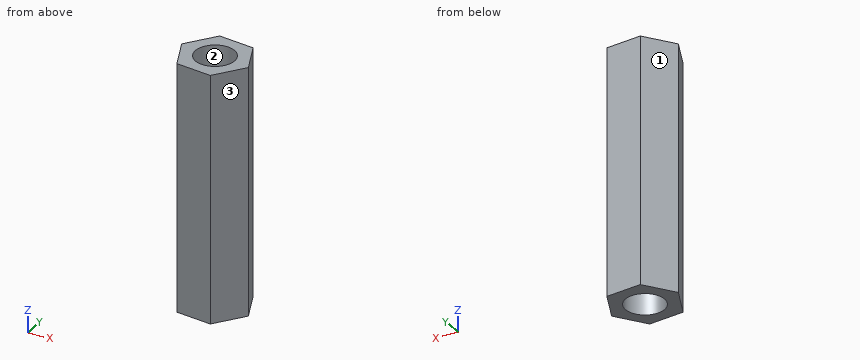
from build123d import *

# Parameters (mm, degrees)
F1_DEPTH = 25
F2_R     = 3.96875
F3_DEPTH = 50.001


with BuildPart() as f1:
    # F0 (on Top) → F1 (new body, symmetric)
    with BuildSketch(Plane.XY):
        Polygon((-2.829355, 6.764472), (-7.272882, 0.931943), (-4.443527, -5.832529), (2.829355, -6.764472), (7.272882, -0.931943), (4.443527, 5.832529), align=None)
    extrude(amount=F1_DEPTH, both=True)

    # F2 (on face) → F3 (cut, through all)
    with BuildSketch(Plane.XY.offset(25)):
        Circle(F2_R)
    extrude(amount=-F3_DEPTH, mode=Mode.SUBTRACT)


solid = f1.part
Could you check a few things on this model? Use its own coordinates, in mm. Face numbers are marked on the shaded views. Round coordinates to 2 decimals unless told otherwise and drop trailing zeros. Write each loop counter-clockwise with the first axis right and the second up, starting at its lowest first coordinate (ties: lowest second). Pieces come first, ordered by that corner, then holes. Notation, with made-up numbers: (23, -36) - (40, -36) arc R18 ccw to (40, -18) - close; hole circle Ø4 at (-6, 10). An arc over 180 degrees is marked (long way). Put each result on its own line as item: value. Start each with the question number.
(1) Thinking about a two-plate mould opening in Y: for the marked faces 1, 2 and 3, which applies, released by +Y, released by -Y, zero draft, split by the parting line, or undercut?
(2) I want a section at B-B, the plane x = -1.5. Please give me the cut outline in (y, z), plus the area to 3 significant figures.
(3) Will these pins go through, and if not, where does the flat tip stop? pin 1 (5 mm diameter, centred on y = 4, z = -16.5, fed in from -X); pin 2 (3 mm diameter, centred on x = 1.5, z = -16, fed in from +Y).
(4) I want a section at C-C, the plane y = 3. Please give me the cut outline in (x, z).
(5) I want a section at A-A, the plane z = -12.5. Please give me the cut outline in (x, y).
(6) I want a section at D-D, the plane x = -5.75. Please give me the cut outline in (y, z), plus the area to 3 significant figures.
(7) I need wall thicknesses on probe 1 along Y at (x, z) = (0, -2); probe 2 along Y at (x, z) = (3.25, -18.5); probe 3 along X at (y, z) = (2.75, -18). Which ranges of each line are inside material? Lowest first, please.
Here are the results:
1. face 1: released by +Y
1. face 2: undercut
1. face 3: released by -Y
2. outline: (-6.21, -25) - (-3.67, -25) - (-3.67, 25) - (-6.21, 25) - close; (3.67, -25) - (6.59, -25) - (6.59, 25) - (3.67, 25) - close
2. area: 273 mm^2
3. pin 1: stops at x = -6.84
3. pin 2: stops at y = 6.4
4. outline: (-5.7, -25) - (-2.6, -25) - (-2.6, 25) - (-5.7, 25) - close; (2.6, -25) - (5.63, -25) - (5.63, 25) - (2.6, 25) - close
5. outline: (-7.27, 0.93) - (-4.44, -5.83) - (2.83, -6.76) - (7.27, -0.93) - (4.44, 5.83) - (-2.83, 6.76) - close; hole circle Ø7.94 at (0, 0)
6. outline: (-2.71, -25) - (2.93, -25) - (2.93, 25) - (-2.71, 25) - close
6. area: 282 mm^2
7. probe 1: y = -6.4 to -3.97, 3.97 to 6.4
7. probe 2: y = -6.21 to -2.28, 2.28 to 5.99
7. probe 3: x = -5.89 to -2.86, 2.86 to 5.73
